Source: CAD feature listing. Evaluate the final solid. Frame: model axes, mm. A direction names the side the tool comes from. Coordinates: 2 decimals unless noted, no trailing zeros. Write each loop counter-clockwise with the first axis right and the second up, starting at its lowest first coordinate (ties: lowest second). Pieces come first, ordered by that corner, then holes. Notation, with made-up numbers: M -21,46.25 L -1,46.25 A13 ccw -1,54.25 Z; hole C -7,63 d8. An arc over 180 degrees is marked long. Write item = value, one per line. Start each with the question number.
1. Section query A-A (x = -31). Output: boundary loops of the cut face in (y, z), then the cut area to 3 significant figures.
2. Section query D-D (x = -35.75). Output: boundary loops of the cut face in (y, z).
3. Pull-direction query (Z, two-part tool) for faces 3 (the face through (-38.6, -0.14, 24.84)), 4 (the face through (-35.6, -0.14, 7.86)), 5 (the face through (-31, 0, 7)), 6 (the face through (-39.5, 0, 15)); classes: pulls with the +Z half, pulls with the -Z half, needs draft (parallel to the pull), parting line crosses it, or undercut.
4. Line query: line 1 along Z through (x, y) = (-32.5, 7.25); line 2 along X through (y, z) = (2, 16); line 3 along Z through (x, y) = (-35.75, -5.75). Output: solid intervals per line, ascending.
5. Access query for faces 1 (the face through (-33, 0, 25.7)), 2 (the face through (-36.5, 0, 15)). Directions: +Z, -Z, +X, -X, +Y, -Y. A direction counts if a zero-diameter tool reaches every point of the face in a straight line with its end or side. Return the directions, or none.
6. Section query C-C (z = 12.25). Output: boundary loops of the cut face in (x, y).
7. Section query B-B (y = 7.75). Output: boundary loops of the cut face in (x, z).
8. Pin query (flat end, axial travel): pin 1 Ø5 at (y, z) = (-0.5, 15) entering from +X; pin 2 Ø5 at (x, z) = (-31, 19.5) entering from +Y; pin 3 Ø2 at (x, y) = (-38.5, 4) entering from -Z. Return the tip coordinate at first contact, or that it passes through.
```python
from build123d import *

# Parameters (mm, degrees)
FILLET_R    = 3
FILLET001_R = 3
FILLET002_R = 3
FILLET003_R = 3


with BuildPart() as part:
    # Sweep: sweep along a path in Sketch005
    with BuildLine(Plane.XY) as sweep_path:
        Line((-30, 10), (-30, -10))
    # Sketch004 → Sweep (sweep)
    with BuildSketch(Plane.XZ):
        Polygon((-29.5, 25.7), (-39.5, 25.7), (-39.5, 4), (-29.5, 4), (-29.5, 7), (-36.5, 7), (-36.5, 22.7), (-29.5, 22.7), align=None)
    sweep(path=sweep_path.line)

    # Fillet
    fillet_edges = [part.edges().sort_by_distance(p)[0] for p in [
        (-39.5, 0, 25.7),
    ]]
    fillet(fillet_edges, radius=FILLET_R)

    # Fillet001
    fillet001_edges = [part.edges().sort_by_distance(p)[0] for p in [
        (-39.5, 0, 4),
    ]]
    fillet(fillet001_edges, radius=FILLET001_R)

    # Fillet002
    fillet002_edges = [part.edges().sort_by_distance(p)[0] for p in [
        (-36.5, 0, 7),
    ]]
    fillet(fillet002_edges, radius=FILLET002_R)

    # Fillet003
    fillet003_edges = [part.edges().sort_by_distance(p)[0] for p in [
        (-36.5, 0, 22.7),
    ]]
    fillet(fillet003_edges, radius=FILLET003_R)


solid = part.part
```
Results are:
q1.outline = M -10,4 L 10,4 L 10,7 L -10,7 Z; M -10,22.7 L 10,22.7 L 10,25.7 L -10,25.7 Z
q1.area = 120 mm^2
q2.outline = M -10,4 L 10,4 L 10,8.02 L -10,8.02 Z; M -10,21.68 L 10,21.68 L 10,25.7 L -10,25.7 Z
q3.face_3 = pulls with the +Z half
q3.face_4 = undercut
q3.face_5 = undercut
q3.face_6 = needs draft
q4.line_1 = 4 to 7, 22.7 to 25.7
q4.line_2 = -39.5 to -36.5
q4.line_3 = 4 to 8.02, 21.68 to 25.7
q5.face_1 = +Z, +X, -X, +Y, -Y
q5.face_2 = +X, +Y, -Y
q6.outline = M -39.5,-10 L -36.5,-10 L -36.5,10 L -39.5,10 Z
q7.outline = M -39.5,7 A3 ccw -36.5,4 L -29.5,4 L -29.5,7 L -33.5,7 A3 cw -36.5,10 L -36.5,19.7 A3 cw -33.5,22.7 L -29.5,22.7 L -29.5,25.7 L -36.5,25.7 A3 ccw -39.5,22.7 Z
q8.pin_1 = -36.5
q8.pin_2 = through
q8.pin_3 = 4.17
